Model file for the job. Use its own axes, mm. A direction names the side the tool comes from. Round coordinates to 2 decimals unless told otherwise and drop trailing zeros. Order: outer loops, then holes, each group sorted by start corner. A loop starts at its lowest first (then second) coordinate and runs counter-clockwise, first axis right, second up. Notation, with made-up numbers: (34, 48.25) - (81, 48.25) arc R26 cw to (81, 77.25) - close; hole circle Ø5 at (-9, -31.75). An arc over 180 degrees is marked (long way). Answer as CSV lines item,"result". Start each with the question number.
1. Pull direction X, two halves, no side cores. Call faces 1 (the face through (195.954, -161.928, 0.093)), 2 (the face through (211.837, -157.215, 0.093)), 3 (the face through (998.368, -166.186, 0.093)): released by +X, released by -X, zero draft, split by the parting line, or undercut.
2. Band-saw the part on B-B on x = 272. List the corners of the cut face in (y, z).
3. Wall check: line 1 along Y through (x, z) = (513, 2); line 2 along X through (y, z) = (-82, 0.5); line 3 along X through (y, z) = (-165, -1). Give the ranges that are in metal, low to high. Write a range as [from, to].
4. Band-saw the part on A-A on z = 2. List the corners of the cut face in (x, y).
5. 3-axis set-ups, long thin cutter, end or side, ignore diameter. For faces 4 (the face through (642, -75, -6.65)), 5 (the face through (504.979, -164.477, 0.093)): which of +Z, -Z, +X, -X, +Y, -Y reach the whole face in a straight line?
6. Band-saw the part on C-C on y = -199. List the corners of the cut face in (x, z).
7. Band-saw the part on D-D on x = 670. List the corners of the cut face in (y, z), then the cut area to 3 significant figures.
8. Pin check, flat tips, straight feed: pin 1 Ø5 at (x, z) = (421.5, -2.5) entering from -Y; pin 2 Ø4 at (y, z) = (-168.5, 3.5) entering from -X; pin 3 Ø12 at (x, y) = (631, -32.5) entering from +Z; pin 4 Ø3 at (y, z) = (-148.5, -2.5) entering from -X. Stop position of each tip, or through.
```python
from build123d import *

# Parameters (mm, degrees)
SKETCH1_W           = 1200
SKETCH1_H           = 13.3
EXTRUDE_THIN1_DEPTH = 6.65
SKETCH2_W           = 400
SKETCH2_H           = 13.3
EXTRUDE_THIN2_DEPTH = 6.65
EXTRUDE_THIN3_DEPTH = 6.65


with BuildPart() as part:
    # Sketch1 → Extrude-Thin1 (new, symmetric)
    with BuildSketch(Plane.XY):
        with Locations((600, -6.65)):
            Rectangle(SKETCH1_W, SKETCH1_H)
    extrude(amount=EXTRUDE_THIN1_DEPTH, both=True)



with BuildPart() as body_2:
    # Sketch2 → Extrude-Thin2 (new, symmetric)
    with BuildSketch(Plane.XY):
        with Locations((600, -306.65)):
            Rectangle(SKETCH2_W, SKETCH2_H)
    extrude(amount=EXTRUDE_THIN2_DEPTH, both=True)


with BuildPart() as part_1:
    add(part.part)

    add(body_2.part)  # Extrude-Thin3 merges body 2
    # Sketch3 → Extrude-Thin3 (add, symmetric)
    with BuildSketch(Plane.XY):
        Polygon((1196.01, -1.33), (801.575558109, -297.155831418), (600, -1.494881561), (398.424441891, -297.155831418), (3.99, -1.33), (-3.99, -11.97), (401.575558109, -316.144168582), (600, -25.105118439), (798.424441891, -316.144168582), (1203.99, -11.97), align=None)
    extrude(amount=EXTRUDE_THIN3_DEPTH, both=True)


solid = part_1.part
```
Reply:
1,face 1,"released by -X"
1,face 2,"undercut"
1,face 3,"released by +X"
2,outline,"(-218.96, -6.65) - (-202.34, -6.65) - (-202.34, 6.65) - (-218.96, 6.65) - close; (-13.3, -6.65) - (0, -6.65) - (0, 6.65) - (-13.3, 6.65) - close"
3,line 1,"y = [-313.3, -300], [-152.71, -129.1], [-13.3, 0]"
3,line 2,"x = [89.38, 111.55], [545.11, 561.21], [638.79, 654.89], [1088.45, 1110.62]"
3,line 3,"x = [200.05, 222.22], [488.53, 504.62], [695.38, 711.47], [977.78, 999.95]"
4,outline,"(-3.99, -11.97) - (401.58, -316.14) - (403.51, -313.3) - (796.49, -313.3) - (798.42, -316.14) - (1203.99, -11.97) - (1200, -6.65) - (1200, 0) - (0, 0) - (0, -6.65) - close; hole (19.95, -13.3) - (398.42, -297.16) - (591.95, -13.3) - close; hole (412.58, -300) - (787.42, -300) - (600, -25.11) - close; hole (608.05, -13.3) - (801.58, -297.16) - (1180.05, -13.3) - close"
5,face 4,"-Z, +X, -X, +Y, -Y"
5,face 5,"+Z, -Z"
6,outline,"(245.38, -6.65) - (267.55, -6.65) - (267.55, 6.65) - (245.38, 6.65) - close; (465.35, -6.65) - (481.44, -6.65) - (481.44, 6.65) - (465.35, 6.65) - close; (718.56, -6.65) - (734.65, -6.65) - (734.65, 6.65) - (718.56, 6.65) - close; (932.45, -6.65) - (954.62, -6.65) - (954.62, 6.65) - (932.45, 6.65) - close"
7,outline,"(-313.3, -6.65) - (-300, -6.65) - (-300, 6.65) - (-313.3, 6.65) - close; (-127.78, -6.65) - (-104.17, -6.65) - (-104.17, 6.65) - (-127.78, 6.65) - close; (-13.3, -6.65) - (0, -6.65) - (0, 6.65) - (-13.3, 6.65) - close"
7,area,"668 mm2"
8,pin 1,"stops at y = -313.3"
8,pin 2,"stops at x = 202.05"
8,pin 3,"passes through"
8,pin 4,"stops at x = 176.05"
